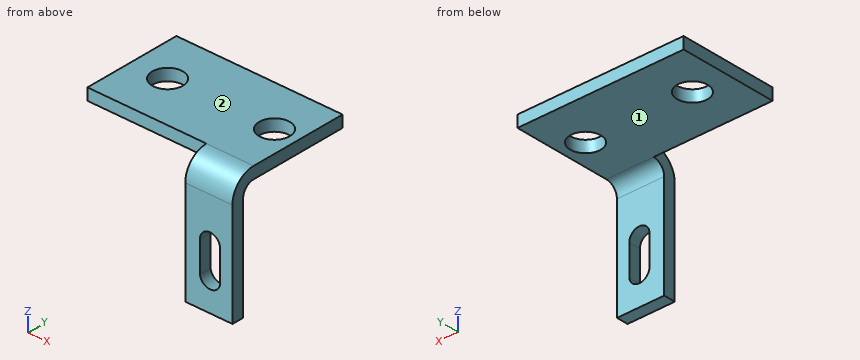
Autodesk Inventor part; units mm, degrees
ref_plane "YZ Plane" through (0, 0, 0) normal (1, 0, 0) x (0, 1, 0)
ref_plane "XZ Plane" through (0, 0, 0) normal (0, 1, 0) x (-1, 0, 0)
ref_plane "XY Plane" through (0, 0, 0) normal (0, 0, 1) x (1, 0, 0)
sketch "Sketch1" plane through (0, 0, 0) normal (0, 1, 0) x (-1, 0, 0)
  line L0 (-3.0226, 8.128) -> (3.0226, 8.128)
  line L1 (3.0226, 8.128) -> (3.0226, -8.128)
  line L2 (3.0226, -8.128) -> (-3.0226, -8.128)
  line L3 (-3.0226, -8.128) -> (-3.0226, 8.128)
  line L4 (-3.0226, 8.128) -> (3.0226, -8.128) construction
  line L5 (3.0226, 8.128) -> (-3.0226, -8.128) construction
  line L6 (1.1394, -0.381) -> (1.1394, -4.3425)
  line L7 (-1.4442, -0.381) -> (-1.4442, -4.3425)
  arc A0 (-1.4442, -4.3425) -> (1.1394, -4.3425) centre (-0.1524, -4.1402) ccw
  arc A1 (1.1394, -0.381) -> (-1.4442, -0.381) centre (-0.1524, -0.381) ccw
  line L8 (0, 9.1418) -> (0, -10.0518)
  point P0 (0, 0)
  dimension "d0" = 16.256
  dimension "d1" = 6.0452
  dimension "d2" = 3.9878
  dimension "d3" = 7.747
  dimension "d4" = 3.175
  dimension "d5" = 3.175
extrude "Plate1" add sketch "Sketch1" along normal blind 1.4986 contours L0 L8 A1 L7 A0 L2 L3 | L0 L1 L2 L8 A0 L6 A1
sketch "Sketch2" plane through (3.0226, 0, 6.6294) normal (0, 0, 1) x (1, 0, 0)
  line L0 (-6.0452, 0) -> (0, 0)
  line L1 (0, 0) -> (0, 15.5956)
  line L2 (0, 15.5956) -> (-6.0452, 15.5956)
  line L3 (-6.0452, 15.5956) -> (-6.0452, 0)
edge flange "Flange1" height 15.5956 angle 90 thickness 1.4986 bend radius 1.4986 thickness toward (0, 0, 1) relief straight relief width 1.4986 relief depth 0.7493 edges at (0, 1.4986, 8.128) wall of the first edge with corners at (-3.0226, 0, 6.6294) (3.0226, 0, 6.6294) (3.0226, 15.5956, 6.6294) (-3.0226, 15.5956, 6.6294)
bend "Bend1"
corner "Corner1"
sketch "Sketch4" plane through (3.0226, 15.5956, 6.6294) normal (0, 0, -1) x (-1, 0, 0)
  circle A0 centre (3.0226, -6.2992) radius 1.9558
  line L0 (6.0452, 0) -> (0, 0)
  point P0 (3.0226, -15.5956)
  dimension "d21" = 6.2992
  dimension "d22" = 3.9116
extrude "Extrusion3" cut sketch "Sketch4" against normal blind 1.4986
sketch "Sketch5" plane through (-3.0226, 15.5956, 6.6294) normal (-1, 0, 0) x (0, 0, 1)
  line L0 (1.4986, -12.5984) -> (1.4986, 0)
  line L1 (0, 0) -> (1.4986, 0)
  line L2 (0, 0) -> (0, -12.5984)
  line L3 (0, -12.5984) -> (1.4986, -12.5984)
  line L4 (0, 0) -> (1.4986, 0)
  line L5 (1.4986, 0) -> (1.4986, -12.5984)
  line L6 (1.4986, -12.5984) -> (0, -12.5984)
  line L7 (0, -12.5984) -> (0, 0)
  point P0 (-6.6294, -15.5956)
extrude "Extrusion4" add sketch "Sketch5" along normal blind 15.24
sketch "Sketch6" plane through (3.0226, 2.9972, 6.6294) normal (0, 0, -1) x (-1, 0, 0)
  circle A0 centre (16.7132, 6.2992) radius 1.9558
  line L0 (21.2852, 12.5984) -> (21.2852, 0)
  line L1 (21.2852, 12.5984) -> (0, 12.5984)
  point P0 (3.0226, -2.9972)
  dimension "d27" = 4.572
  dimension "d28" = 6.2992
  dimension "d29" = 3.9116
extrude "Extrusion5" cut sketch "Sketch6" against normal up to surface (1.4986 mm away)
equation "\"d11\" = BendReliefWidth"
equation "\"d12\" = BendReliefDepth"
equation "\"d13\" = MinimumRemnant"
equation "\"d14\" = BendRadius"
equation "\"d17\" = BendRadius"
equation "\"d18\" = CornerReliefSize"
equation "\"d19\" = GapSize"
equation "\"d20\" = JacobiRadiusSize"
equation "\"BendRadius\" = Thickness"
equation "\"BendReliefWidth\" = Thickness"
equation "\"BendReliefDepth\" = 0.5 * Thickness"
equation "\"CornerReliefSize\" = 4 * Thickness"
equation "\"MinimumRemnant\" = 2 * Thickness"
equation "\"TransitionRadius\" = BendRadius"
equation "\"JacobiRadiusSize\" = Thickness"
equation "\"GapSize\" = Thickness"
equation "\"d10\" = BendRadius"
properties part number "dsub37Bracket_right"
Input: part model. Units: mm. Frame: model coordinates. Face numbers are marked on the shaded views. A direction names the side the tool comes from. Give positions to 0.01 mm unless a question says otherwise; leave off trailing zeros. Order: outer loops, then holes, each group sorted by start corner. A loop starts at its lowest first (then second) coordinate and runs counter-clockwise, first axis right, second up.
Q1. Section B-B on x = -15.25. Output: boundary loops of the cut face in (y, z), and give its area (3 significant figures).
Checked values:
outline: (3, 6.63) - (8.12, 6.63) - (8.12, 8.13) - (3, 8.13) - close; (10.48, 6.63) - (15.6, 6.63) - (15.6, 8.13) - (10.48, 8.13) - close
area: 15.3 mm2
Q2. Section D-D on y = 12.75. Output: boundary loops of the cut face in (x, z), and give its area (3 significant figures).
Checked values:
outline: (-18.26, 6.63) - (3.02, 6.63) - (3.02, 8.13) - (-18.26, 8.13) - close
area: 31.9 mm2
Q3. Set-up query: the marked faces 1 and 2. Return all of +Z, -Z, +X, -X, +Y, -Y with unobstructed straight access to the full face (end or side cutting, diameter ignored); none if empty.
Checked values:
face 1: -Z, +X, -X, +Y
face 2: +Z, +X, -X, +Y, -Y
Q4. Contact query for flat-ended pins moving along their axis: pin 1 Ø2 at (x, y) = (-1.5, 6.5) entering from -Z; pin 2 Ø1.2 at (x, z) = (-8, 7) entering from -Y; pin 3 Ø2.5 at (y, z) = (1.5, -2.5) entering from -X. Output: stop coordinate, or through.
Checked values:
pin 1: stops at z = 6.63
pin 2: stops at y = 3
pin 3: stops at x = -3.02
Q5. Section C-C on x = 0. Output: boundary loops of the cut face in (y, z), and give its area (3 significant figures).
Checked values:
outline: (0, -8.13) - (1.5, -8.13) - (1.5, -5.44) - (0, -5.44) - close; (0, 0.9) - (1.5, 0.9) - (1.5, 5.13) arc R1.5 cw to (3, 6.63) - (7.34, 6.63) - (7.34, 8.13) - (3, 8.13) arc R3 ccw to (0, 5.13) - close; (11.25, 6.63) - (15.6, 6.63) - (15.6, 8.13) - (11.25, 8.13) - close
area: 28.7 mm2
Q6. Section A-A on z = -3.25. Output: boundary loops of the cut face in (x, y), and give its area (3 significant figures).
Checked values:
outline: (-3.02, 0) - (-1.14, 0) - (-1.14, 1.5) - (-3.02, 1.5) - close; (1.44, 0) - (3.02, 0) - (3.02, 1.5) - (1.44, 1.5) - close
area: 5.19 mm2
Q7. Ray query, probe 1 along Z at (x, y) = (-1.25, 7.75); probe 2 along X at (y, z) = (9.5, 7.25); probe 3 along Y at (x, z) = (0, 7.5). Return the intervals inside material, ascending.
Checked values:
probe 1: z = 6.63 to 8.13
probe 2: x = -18.26 to -15.64, -11.75 to -1.95, 1.95 to 3.02
probe 3: y = 1.16 to 7.34, 11.25 to 15.6
